Autodesk Inventor part; units mm, degrees
ref_plane "YZ Plane" through (0, 0, 0) normal (1, 0, 0) x (0, 1, 0)
ref_plane "XZ Plane" through (0, 0, 0) normal (0, 1, 0) x (-1, 0, 0)
ref_plane "XY Plane" through (0, 0, 0) normal (0, 0, 1) x (1, 0, 0)
sketch "Sketch1" plane through (0, 0, 0) normal (0, 1, 0) x (-1, 0, 0)
  arc A0 (2, 1.5) -> (2, -1.5) centre (0, 0) ccw
  line L0 (2, 0) -> (2, -1.5)
  line L1 (2, 0) -> (2, 1.5)
sketch "Sketch1 outline for Extrusion1" plane through (0, 0, 0) normal (0, 1, 0) x (-1, 0, 0)
  line L0 (2, 0) -> (2, -1.5)
  arc A0 (2, -1.5) -> (2, 1.5) centre (0, 0) cw
  line L1 (2, 1.5) -> (2, 0)
extrude "Extrusion1" add sketch "Sketch1 outline for Extrusion1" along normal blind 22
thicken "Thicken1" operation add thickness 1 both sides no extend neighbours yes toward (-0.5598596, 0, 0.8285875) faces at (-1.399649, 14.666667, 2.071469) (-2, 14.666667, -0.5) (-2, 14.666667, 1)
sketch "Sketch2" plane through (0, 22, 0) normal (0, 1, 0) x (1, 0, 0)
  arc A0 (-2, -1.813836) -> (-2, 1.813836) centre (0, 0) ccw
  line L0 (-2, 0) -> (-2, 1.813836)
  line L1 (-2, 0) -> (-2, -1.813836)
  dimension "d8" = 5.4
sketch "Sketch2 outline for Extrusion2" plane through (0, 22, 0) normal (0, 1, 0) x (1, 0, 0)
  line L0 (-2, 0) -> (-2, 1.813836)
  arc A0 (-2, 1.813836) -> (-2, -1.813836) centre (0, 0) cw
  line L1 (-2, -1.813836) -> (-2, 0)
extrude "Extrusion2" cut sketch "Sketch2 outline for Extrusion2" against normal blind 22
sketch "Sketch3" plane through (0, 22, 0) normal (0, 1, 0) x (1, 0, 0)
  arc A0 (-3, -1.802776) -> (-3, 1.802776) centre (0, 0) ccw
  line L0 (-3, -1.802776) -> (-3, 2.552776)
  line L1 (-3, 2.552776) -> (-1.3277, 3.238397)
  line L2 (-3, -1.802776) -> (-3, -2.552776)
  line L3 (-3, -2.552776) -> (-1.3277, -3.238397)
  line L4 (-1.3277, -3.238397) -> (-2, -1.813836)
  line L5 (-2, 1.813836) -> (-2, -1.813836)
  line L6 (-2, -1.813836) -> (-2, 1.813836)
  line L7 (-2, 1.813836) -> (-1.3277, 3.238397)
  dimension "d12" = 4.35555
  dimension "d13" = 0.75
sketch "Sketch3 outline for Extrusion3" plane through (0, 22, 0) normal (0, 1, 0) x (1, 0, 0)
  line L0 (-3, -2.552776) -> (-1.3277, -3.238397)
  line L1 (-1.3277, -3.238397) -> (-2, -1.813836)
  line L2 (-2, -1.813836) -> (-2, 1.813836)
  line L3 (-2, 1.813836) -> (-1.3277, 3.238397)
  line L4 (-1.3277, 3.238397) -> (-3, 2.552776)
  line L5 (-3, 2.552776) -> (-3, -2.552776)
extrude "Extrusion3" add sketch "Sketch3 outline for Extrusion3" against normal blind 22
properties part number "MirrorMount"
Here's how the part is built. I have some questions about the finished solid (model axes, mm). Coordinates: 2 decimals unless noted, no trailing zeros. Order: outer loops, then holes, each group sorted by start corner. A loop starts at its lowest first (then second) coordinate and runs counter-clockwise, first axis right, second up.
Item 1: If we section it at C-C on y = 10.75: List the corners of the cut face in (x, z) for me, plus the area to 3 significant figures.
Result sheet:
outline: (-3, -2.55) - (-1.33, -3.24) arc R3.5 ccw (long way) to (-1.33, 3.24) - (-3, 2.55) - close; hole (-2, -1.81) arc R2.7 ccw (long way) to (-2, 1.81) - close
area: 16.8 mm2
Item 2: I need wall thicknesses on line 1 (Z direction, x = 0, y = 14); line 2 (X direction, y = 14.5, z = -1.25); line 3 (Z direction, x = 1, y = 3.75). Which ranges of each line are inside material? Lowest first, please.
Result sheet:
line 1: z = -3.5 to -2.7, 2.7 to 3.5
line 2: x = -3 to -2, 2.39 to 3.27
line 3: z = -3.35 to -2.51, 2.51 to 3.35
Item 3: For P1, Ø1, axis at x = 1, y = 15.5, coming from the -Z side; P2, Ø1, axis at x = 2.5, y = 10, coming from the -Z side, each with a flat end and sliding along its axis, tell me the tip position at first contact or that it passes through.
Result sheet:
P1: stops at z = -3.46
P2: stops at z = -2.87
Item 4: If we section it at B-B on x = 0: List the corners of the cut face in (y, z) for me, plus the area to 3 significant figures.
Result sheet:
outline: (0, -3.5) - (22, -3.5) - (22, -2.7) - (0, -2.7) - close; (0, 2.7) - (22, 2.7) - (22, 3.5) - (0, 3.5) - close
area: 35.2 mm2
Item 5: If we section it at A-A on z = 0: List the corners of the cut face in (x, y) for me.
Result sheet:
outline: (-3, 0) - (-2, 0) - (-2, 22) - (-3, 22) - close; (2.7, 0) - (3.5, 0) - (3.5, 22) - (2.7, 22) - close
Item 6: If we mould it in two halves opening along X, with no side actions, what happens to faces 1 (the face through (-2.15, 11.15, -2.9)), 2 (the face through (-2, 11, 0)), 3 (the face through (-2.2, 22, 0))? For each: +X half, -X half, draft (parallel to the pull), parting line (faces both ways), or undercut.
Result sheet:
face 1: -X half
face 2: undercut
face 3: draft
